Source: CAD feature listing. Evaluate the final solid. Frame: model axes, mm. Face numbers are marked on the shaded views. A direction names the side the tool comes from. Give positions to 0.01 mm unless a question says otherwise; leave off trailing zeros. Order: outer loops, then holes, each group sorted by start corner. A loop starts at its lowest first (then second) coordinate and runs counter-clockwise, first axis right, second up. Notation, with made-up numbers: M 13.5,37.5 L 66.5,37.5 A16 ccw 66.5,62.5 Z; hole C 54.25,59.5 d1. An arc over 180 degrees is marked long. Answer in a Markdown table with one row per item. Add a question column.
(1) Section query A-A, the plane x = -7.5. Return loops of the section in (y, z).
(2) Section query C-C, the plane x = 0. Return loops of the section in (y, z), plus the area to 3 significant figures.
(3) Pin query (flat end, axial travel): P1, Ø0.8, axis at y = -5, z = 8.5, coming from the +X side; P2, Ø4, axis at x = 22, y = -9, coming from the +Z side; P3, Ø1.8, axis at x = 28, y = 8, coming from the +Z side; P4, Ø7, axis at y = 0, z = 9, coming from the -X side. Return the tip coordinate at first contact, or that it passes through.
(4) Set-up query: the marked faces 4, 5 and 6. Return all of +Z, -Z, +X, -X, +Y, -Y with unobstructed straight access to the full face (end or side cutting, diameter ignored); none if empty.
(5) Section query D-D, the plane z = 9. Count the separate pieces of the cut face and the enclosed holes in it, plus the area to 3 significant figures.
(6) Material intervals for line 1 along Y through (x, z) = (-28, 9); line 2 along Y through (x, z) = (38.55, 9); line 3 along Y through (x, z) = (0, 16.5), sorted ascending.
(7) Section query B-B, the plane y = -13. Return loops of the section in (x, z), plus the area to 3 significant figures.
(8) Mould query, pull axis Z, two halves, no side actions, for the marked faces 1, 2 and 3. Classes: pulls with the +Z half, pulls with the -Z half, needs draft (parallel to the pull), parting line crosses it, or undercut.
from build123d import *

# Parameters (mm, degrees)
SKETCH2_W           = 68
SKETCH2_H           = 32
BOSS_EXTRUDE1_DEPTH = 18
SKETCH3_R           = 8
BOSS_EXTRUDE2_DEPTH = 6
FILLET1_R           = 1
SKETCH4_R           = 4
CUT_EXTRUDE1_DEPTH  = 10
CUT_EXTRUDE2_DEPTH  = 47.69047012
SKETCH6_R           = 1.5
CUT_EXTRUDE3_DEPTH  = 47.69047012
SKETCH7_R           = 3.5
CUT_EXTRUDE4_DEPTH  = 12
SKETCH8_R           = 3
CUT_EXTRUDE5_DEPTH  = 67.513156593
SKETCH9_R           = 1.25
CUT_EXTRUDE6_DEPTH  = 5
SKETCH10_R          = 4
SKETCH10_R_2        = 1.5
CUT_EXTRUDE9_DEPTH  = 47.69047012
CHAMFER1_SIZE       = 0.5
CHAMFER2_SIZE       = 0.5


with BuildPart() as part:
    # Sketch2 → Boss-Extrude1 (new body)
    with BuildSketch(Plane.XY):
        Rectangle(SKETCH2_W, SKETCH2_H)
    extrude(amount=BOSS_EXTRUDE1_DEPTH)

    # Sketch3 → Boss-Extrude2 (add)
    with BuildSketch(Plane(origin=(34, 0, 0), x_dir=(0, 0, -1), z_dir=(1, 0, 0))):
        with Locations((-9, 0)):
            Circle(SKETCH3_R)
    extrude(amount=BOSS_EXTRUDE2_DEPTH)

    # Fillet1
    fillet1_edges = [part.edges().sort_by_distance(p)[0] for p in [
        (34, 0, 17),
    ]]
    fillet(fillet1_edges, radius=FILLET1_R - 0.0001)  # a hair under: the kernel refuses the full size

    # Sketch4 → Cut-Extrude1 (cut)
    with BuildSketch(Plane.ZY.offset(34)):
        with Locations((9, 0)):
            Circle(SKETCH4_R)
    extrude(amount=-CUT_EXTRUDE1_DEPTH, mode=Mode.SUBTRACT)

    # Sketch5 → Cut-Extrude2 (cut, through all)
    with BuildSketch(Plane.XY.offset(18)):
        with BuildLine():
            Line((22, -10), (-22, -10))
            ThreePointArc((-22, -10), (-23.414213562, -9.414213562), (-24, -8))
            Line((-24, -8), (-24, 8))
            ThreePointArc((-24, 8), (-23.414213562, 9.414213562), (-22, 10))
            Line((-22, 10), (22, 10))
            ThreePointArc((22, 10), (23.414213562, 9.414213562), (24, 8))
            Line((24, 8), (24, -8))
            ThreePointArc((24, -8), (23.414213562, -9.414213562), (22, -10))
        make_face()
    extrude(amount=-CUT_EXTRUDE2_DEPTH, mode=Mode.SUBTRACT)

    # Sketch6 → Cut-Extrude3 (cut, through all)
    with BuildSketch(Plane.XY.offset(18)):
        with Locations((-22.5, 13)):
            Circle(SKETCH6_R)
        with Locations((-7.5, 13)):
            Circle(SKETCH6_R)
        with Locations((7.5, 13)):
            Circle(SKETCH6_R)
        with Locations((22.5, 13)):
            Circle(SKETCH6_R)
        with Locations(Location((22.5, -13, 0), (0, 0, 180))):
            Circle(SKETCH6_R)
        with Locations(Location((7.5, -13, 0), (0, 0, 180))):
            Circle(SKETCH6_R)
        with Locations(Location((-7.5, -13, 0), (0, 0, 180))):
            Circle(SKETCH6_R)
        with Locations(Location((-22.5, -13, 0), (0, 0, 180))):
            Circle(SKETCH6_R)
        with Locations((28, -8)):
            Circle(SKETCH6_R)
        with Locations(Location((28, 8, 0), (0, 0, 180))):
            Circle(SKETCH6_R)
        with Locations((-28, 8)):
            Circle(SKETCH6_R)
        with Locations(Location((-28, -8, 0), (0, 0, 180))):
            Circle(SKETCH6_R)
    extrude(amount=-CUT_EXTRUDE3_DEPTH, mode=Mode.SUBTRACT)

    # Sketch7 → Cut-Extrude4 (cut)
    with BuildSketch(Plane(origin=(40, 0, 0), x_dir=(0, 0, -1), z_dir=(1, 0, 0))):
        with Locations((-9, 0)):
            Circle(SKETCH7_R)
    extrude(amount=-CUT_EXTRUDE4_DEPTH, mode=Mode.SUBTRACT)

    # Sketch8 → Cut-Extrude5 (cut, through all)
    with BuildSketch(Plane(origin=(28, 0, 0), x_dir=(0, 0, -1), z_dir=(1, 0, 0))):
        with Locations((-9, 0)):
            Circle(SKETCH8_R)
    extrude(amount=-CUT_EXTRUDE5_DEPTH, mode=Mode.SUBTRACT)

    # Sketch9 → Cut-Extrude6 (cut)
    with BuildSketch(Plane(origin=(40, 0, 0), x_dir=(0, 0, -1), z_dir=(1, 0, 0))):
        with Locations((-9, 5.5)):
            Circle(SKETCH9_R)
        with Locations((-9, -5.5)):
            Circle(SKETCH9_R)
        with Locations((-3.5, 0)):
            Circle(SKETCH9_R)
        with Locations((-14.5, 0)):
            Circle(SKETCH9_R)
    extrude(amount=-CUT_EXTRUDE6_DEPTH, mode=Mode.SUBTRACT)

    # Sketch10 → Cut-Extrude9 (cut, through all)
    with BuildSketch(Plane(origin=(0, 0, 0), x_dir=(1, 0, 0), z_dir=(0, 1, 0))):
        with Locations(Location((0, -9, 0), (0, 0, 180))):
            Circle(SKETCH10_R)
        with Locations(Location((-11, -4, 0), (0, 0, 180))):
            Circle(SKETCH10_R_2)
        with Locations(Location((11, -4, 0), (0, 0, 90))):
            Circle(SKETCH10_R_2)
        with Locations(Location((11, -14, 0), (0, 0, 180))):
            Circle(SKETCH10_R_2)
        with Locations(Location((-11, -14, 0), (0, 0, 90))):
            Circle(SKETCH10_R_2)
    extrude(amount=CUT_EXTRUDE9_DEPTH, mode=Mode.SUBTRACT)

    # Chamfer1
    chamfer1_edges = [part.edges().sort_by_distance(p)[0] for p in [
        (-34, 0, 5),
    ]]
    chamfer(chamfer1_edges, length=CHAMFER1_SIZE)

    # Chamfer2
    chamfer2_edges = [part.edges().sort_by_distance(p)[0] for p in [
        (40, 0, 12.5),
        (40, 0, 17),
    ]]
    chamfer(chamfer2_edges, length=CHAMFER2_SIZE)


solid = part.part
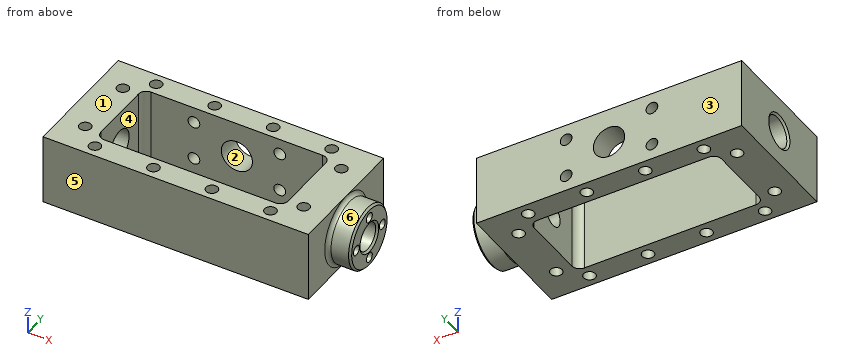
Values follow:
| question | item | result |
|---|---|---|
| 1 | outline | M -16,0 L -14.5,0 L -14.5,18 L -16,18 Z; M -11.5,0 L -10,0 L -10,18 L -11.5,18 Z; M 10,0 L 11.5,0 L 11.5,18 L 10,18 Z; M 14.5,0 L 16,0 L 16,18 L 14.5,18 Z |
| 2 | outline | M -16,0 L -10,0 L -10,18 L -16,18 Z; M 10,0 L 16,0 L 16,5 L 10,5 Z; M 10,13 L 16,13 L 16,18 L 10,18 Z |
| 2 | area | 168 mm² |
| 3 | P1 | stops at x = 35 |
| 3 | P2 | stops at z = 18 |
| 3 | P3 | passes through |
| 3 | P4 | stops at x = 24 |
| 4 | face 4 | +Z, -Z |
| 4 | face 5 | +Z, -Z, +X, -X, -Y |
| 4 | face 6 | +X |
| 5 | separate pieces | 3 |
| 5 | enclosed holes | 12 |
| 5 | area | 969 mm² |
| 6 | line 1 | y = -16 to -9.5, -6.5 to -4, 4 to 6.5, 9.5 to 16 |
| 6 | line 2 | y = -8 to -6.75, -4.25 to -3.5, 3.5 to 4.25, 6.75 to 8 |
| 6 | line 3 | y = -16 to -10, 10 to 16 |
| 7 | outline | M -34,0 L -24,0 L -24,18 L -34,18 Z; M -21,0 L -9,0 L -9,18 L -21,18 Z; M -6,0 L 6,0 L 6,18 L -6,18 Z; M 9,0 L 21,0 L 21,18 L 9,18 Z; M 24,0 L 34,0 L 34,18 L 24,18 Z |
| 7 | area | 1,010 mm² |
| 8 | face 1 | pulls with the +Z half |
| 8 | face 2 | undercut |
| 8 | face 3 | needs draft |
